from build123d import *

# Parameters (mm, degrees)
F0_R     = 19.05
F1_DEPTH = 50.8
F0_R_2   = 9.525
F2_DEPTH = 19.05
F0_R_3   = 12.7
F3_DEPTH = 34.544


with BuildPart() as f1:
    # F0 (on Front) → F1 (new body)
    with BuildSketch(Plane.XZ):
        with BuildLine():
            ThreePointArc((29.100271, -12.697902), (31.080509, -6.485711), (31.75, 0))
            ThreePointArc((31.75, 0), (31.080718, 6.484712), (29.101087, 12.696032))
            ThreePointArc((29.101087, 12.696032), (0.001961, 31.75), (-29.099518, 12.699628))
            ThreePointArc((-29.099518, 12.699628), (-31.749679, 0.142707), (-29.212504, -12.437529))
            ThreePointArc((-29.212504, -12.437529), (-0.141766, -31.749684), (29.100271, -12.697902))
        make_face()
        Circle(F0_R, mode=Mode.SUBTRACT)
    extrude(amount=F1_DEPTH)

    # F0 (on Front) → F2 (join)
    with BuildSketch(Plane.XZ):
        with BuildLine():
            ThreePointArc((-29.212504, -12.437529), (-31.749679, 0.142707), (-29.099518, 12.699628))
            Line((-29.099518, 12.699628), (-50.702789, 12.699628))
            Line((-50.702789, 12.699628), (-50.897211, 12.699628))
            ThreePointArc((-50.897211, 12.699628), (-63.499374, -0.126084), (-50.645043, -12.699055))
            Line((-50.645043, -12.699055), (-29.212504, -12.437529))
        make_face()
        with Locations((-44.891737, 0)):
            Circle(F0_R_2, mode=Mode.SUBTRACT)
        with BuildLine():
            ThreePointArc((29.101087, 12.696032), (31.080718, 6.484712), (31.75, 0))
            ThreePointArc((31.75, 0), (31.080509, -6.485711), (29.100271, -12.697902))
            Line((29.100271, -12.697902), (85.367147, -12.697902))
            Line((85.367147, -12.697902), (85.828853, -12.697902))
            ThreePointArc((85.828853, -12.697902), (98.295041, 0.274142), (85.280573, 12.696032))
            Line((85.280573, 12.696032), (29.101087, 12.696032))
        make_face()
        with BuildLine():
            ThreePointArc((45.121247, -9.508264), (35.988966, -0.012772), (45.095725, 9.5072))
            Line((45.095725, 9.5072), (80.063554, 9.524999))
            ThreePointArc((80.063554, 9.524999), (89.589145, 0.284741), (80.63279, -9.508264))
            ThreePointArc((80.63279, -9.508264), (80.068402, -9.525), (79.504014, -9.508264))
            Line((79.504014, -9.508264), (45.888676, -9.508264))
            ThreePointArc((45.888676, -9.508264), (45.504961, -9.516004), (45.121247, -9.508264))
        make_face(mode=Mode.SUBTRACT)
    extrude(amount=F2_DEPTH)

    # F0 (on Front) → F3 (join)
    with BuildSketch(Plane.XZ):
        Circle(F0_R)
        Circle(F0_R_3, mode=Mode.SUBTRACT)
    extrude(amount=F3_DEPTH)


solid = f1.part
Work out the finished part from the listing and answer in its coordinate system (mm). A direction names the side the tool comes from. Coordinates: 2 decimals unless noted, no trailing zeros. Loops run counter-clockwise (first coordinate to the right, second up) from the corner with the lowest first, then second, coordinate; pieces in that order, holes last. Notation, with made-up numbers: (-1, 6.5) -> (38, 6.5) arc R10 ccw to (38, 25.5) -> close; hole circle Ø9 at (71.5, -10.75). An arc over 180 degrees is marked (long way). Write each question's results on one line, items separated by ' | '. Start each with the question number.
1) Find section C-C on x = 0. Determine the outline of the cut face in (y, z).
2) Find section A-A on y = -12. Count the separate pieces of the cut face and the enclosed holes in it, then the cut area to 3 significant figures.
3) For faces 1 (the cylindrical face through (-15.12, -42.56, -11.59)), 2 (the flat face through (63, -9, -9.508)), 3 (the flat face through (-40, -9, 12.7)), 4 (the flat face through (58, -9, 12.696)), 5 (the flat face through (57, -9, -12.698)), determine the directions among +Z, -Z, +X, -X, +Y, -Y from which every point of the face is accessible in a straight line to the end or side of a thin tool.
4) Find section D-D on y = -31.5. Determine the outline of the cut face in (x, z), then the cut area to 3 significant figures.
5) The mould has two halves that part along X. Classify faces 6 (the cylindrical face through (35.99, -9.39, -0.22)), 7 (the cylindrical face through (31.1, -34.7, 6.4)), 8 (the cylindrical face through (89.58, -9.39, 0.49)), 9 (the flat face through (-54.2, -19.05, 3)): pulls with the +X half, pulls with the -X half, needs draft (parallel to the pull), parting line crosses it, or undercut.
6) Consider line 1 along X through (y, z) = (-23.5, 0.5); line 2 along Z through (x, y) = (0, -26); line 3 along X through (y, z) = (-7.5, -1). Determine where each line is inside the solid, lowest interval first.
7) Flat-ended cylindrical pins translate along their axes: P1, Ø12, axis at x = -9.5, z = -6, coming from the -Y side; P2, Ø20.5, axis at x = 68.5, z = -5, coming from the -Y side; P3, Ø9.5, axis at x = 67, y = -6.5, coming from the +Z side. Find the tip coordinate at first contact, or state that the pin passes through.
8) Find section B-B on z = -7. Determine the outline of the cut face in (x, y).
Response values:
1) outline: (-50.8, -31.75) -> (0, -31.75) -> (0, -12.7) -> (-34.54, -12.7) -> (-34.54, -19.05) -> (-50.8, -19.05) -> close; (-50.8, 19.05) -> (-34.54, 19.05) -> (-34.54, 12.7) -> (0, 12.7) -> (0, 31.75) -> (-50.8, 31.75) -> close
2) separate pieces: 1 | enclosed holes: 3 | area: 3,830 mm^2
3) face 1: -Y | face 2: +Y, -Y | face 3: +Z, -X, +Y, -Y | face 4: +Z, +X, +Y, -Y | face 5: -Z, +X, +Y, -Y
4) outline: (-29.21, -12.44) arc R31.75 ccw to (29.1, -12.7) arc R31.75 ccw to (31.75, 0) arc R31.75 ccw to (29.1, 12.7) arc R31.75 ccw to (-29.1, 12.7) arc R31.75 ccw to start; hole circle Ø25.4 at (0, 0) | area: 2,660 mm^2
5) face 6: undercut | face 7: pulls with the +X half | face 8: undercut | face 9: needs draft
6) line 1: x = -31.75 to -12.69, 12.69 to 31.75 | line 2: z = -31.75 to -12.7, 12.7 to 31.75 | line 3: x = -63.46 to -54.36, -35.42 to -12.66, 12.66 to 36.04, 89.54 to 98.26
7) P1: stops at y = -34.54 | P2: stops at y = -19.05 | P3: stops at z = 12.7
8) outline: (-61.4, -19.05) -> (-51.35, -19.05) -> (-51.35, 0) -> (-61.4, 0) -> close; (-38.43, -19.05) -> (-30.97, -19.05) -> (-30.97, -50.8) -> (-17.72, -50.8) -> (-17.72, -34.54) -> (-10.6, -34.54) -> (-10.6, 0) -> (-38.43, 0) -> close; (10.6, -34.54) -> (17.72, -34.54) -> (17.72, -50.8) -> (30.97, -50.8) -> (30.97, -19.05) -> (39.06, -19.05) -> (39.06, 0) -> (10.6, 0) -> close; (86.53, -19.05) -> (96.19, -19.05) -> (96.19, 0) -> (86.53, 0) -> close
